Could you check a few things on this model? Use its own coordinates, in mm. Give positions to 0.01 mm unless a question says otherwise; leave off trailing zeros. Loops run counter-clockwise (first coordinate to the right, second up) from the corner with the lowest first, then second, coordinate; pieces in that order, holes last. Notation, with made-up numbers: (60.25, -26) -> (89.25, -26) arc R28 cw to (89.25, -1) -> close; hole circle Ø8 at (-11.75, -22). An arc over 180 degrees is marked (long way). Write item = value, one per line. Start each with the question number.
1) If we mould it in two halves opening along X, with no side actions, what happens to faces 1 (the face through (1.617, 0.67, 4.447)), 2 (the face through (-1.08, 4.88, 4.48))? For each: +X half, -X half, draft (parallel to the pull), parting line (faces both ways), or undercut.
2) I'm going to push a flat-ended pin straight in: pin 1 Ø1.5 at (x, z) = (-4, 2.5) entering from +Y. Where does the tip first touch, or does it pass through?
3) I want a section at A-A (z = 4.75). List the corners of the cut face in (x, y) for me, and give its area (3 significant figures).
4) I need wall thicknesses on probe 1 along X at (y, z) = (0, 3.25); probe 2 along Y at (x, z) = (0, 6.5). Which ranges of each line are inside material? Lowest first, please. Write a range as from..to.
Autodesk Inventor part; units mm, degrees
ref_plane "YZ Plane" through (0, 0, 0) normal (1, 0, 0) x (0, 1, 0)
ref_plane "XZ Plane" through (0, 0, 0) normal (0, 1, 0) x (-1, 0, 0)
ref_plane "XY Plane" through (0, 0, 0) normal (0, 0, 1) x (1, 0, 0)
sketch "Sketch1" plane through (0, 0, 0) normal (0, 0, 1) x (1, 0, 0)
  circle A0 centre (0, 0) radius 5
  dimension "d0" = 10
extrude "Extrusion1" add sketch "Sketch1" along normal blind 9
chamfer "Chamfer1" distance 5 distance2 2 1 edges at (-5, 0, 9) measured on face at (-0.591, 1.5584, 9)
chamfer "Chamfer2" distance 2 distance2 5 1 edges at (-5, 0, 0) measured on face at (4.9838, -0.4023, 4.6667)
sketch "Sketch3" plane through (0, 0, 0) normal (0, 0, 1) x (1, 0, 0)
  circle A0 centre (0, 0) radius 1.75
  dimension "d11" = 3.5
extrude "Extrusion2" cut sketch "Sketch3" along normal blind 10
fillet "Fillet1" radius 2 2 edges at (-5, 0, 2) (-5, 0, 7)
properties part number "KoloPrzegubu"
Answer list:
q1.face_1 = undercut
q1.face_2 = parting line
q2.pin_1 = 3.64
q3.outline = circle Ø10 at (0, 0); hole circle Ø3.5 at (0, 0)
q3.area = 68.9 mm^2
q4.probe_1 = -5..-1.75, 1.75..5
q4.probe_2 = -4.81..-1.75, 1.75..4.81
